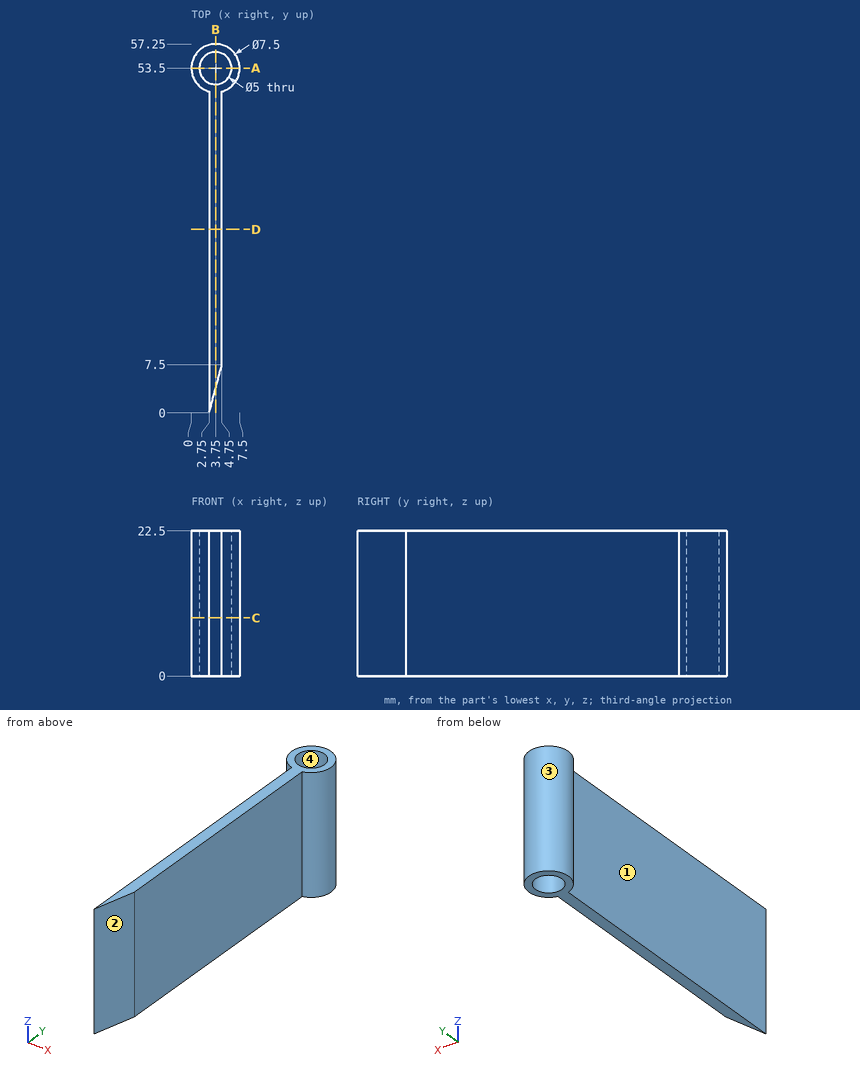
Print and shaded views of the part. All mm, measured from the part's lowest x, y and z. Round coordinates to 2 decimals unless told otherwise and drop trailing zeros. Write each loop counter-clockwise with the first axis right and the second up, starting at its lowest first coordinate (ties: lowest second). Pieces come first, ordered by that corner, then holes. Notation, with made-up numbers: (6.25, 67.25) - (40.25, 67.25) arc R23 ccw to (40.25, 98.25) - close; hole circle Ø5 at (0.5, 74.25). An arc over 180 degrees is marked (long way). Use CSV: the item, a comma, the result in double quotes. Start each with the question number.
Item 1: Two-plate mould, pull along Y, no slides. Class the marked faces 1, 2, 3 and 4: released by +Y, released by -Y, zero draft, split by the parting line, or undercut.
Item 2: Pin check, flat tips, straight feed: P1, Ø4, axis at y = 7, z = 18, coming from the +X side; P2, Ø1, axis at y = 29.5, z = 9.5, coming from the -X side; P3, Ø2, axis at y = 51.5, z = 3.5, coming from the -X side. Stop position of each tip, or through.
Item 3: Band-saw the part on D-D (y = 28.5). Write the cut outline in (x, z), and give its area (3 significant figures).
Item 4: Band-saw the part on C-C (z = 9). Write the cut outline in (x, y).
Item 5: Drill centre lines: L1, parallel to X at y = 48.5, z = 7; L2, parallel to Y at x = 2.5, z = 8; L3, parallel to Y at x = 5.75, z = 19.5. Where is each one in solid material? Low to high. Write a range as [from, to].
Item 6: Band-saw the part on B-B (x = 3.75). Write the cut outline in (y, z).
Item 7: Band-saw the part on A-A (y = 53.5). Write the cut outline in (x, z), and give its area (4 significant figures).
Checked values:
1,face 1,"zero draft"
1,face 2,"released by -Y"
1,face 3,"split by the parting line"
1,face 4,"undercut"
2,P1,"stops at x = 4.75"
2,P2,"stops at x = 2.75"
2,P3,"stops at x = 0.14"
3,outline,"(2.75, 0) - (4.75, 0) - (4.75, 22.5) - (2.75, 22.5) - close"
3,area,"45.0 mm²"
4,outline,"(2.75, 0) - (4.75, 7.5) - (4.75, 49.89) arc R3.75 ccw (long way) to (2.75, 49.89) - close; hole circle Ø5 at (3.75, 53.5)"
5,L1,"x = [2.75, 4.75]"
5,L2,"y = [49.96, 51.33], [55.67, 57.04]"
5,L3,"y = [50.33, 52], [55, 56.67]"
6,outline,"(3.75, 0) - (51, 0) - (51, 22.5) - (3.75, 22.5) - close; (56, 0) - (57.25, 0) - (57.25, 22.5) - (56, 22.5) - close"
7,outline,"(0, 0) - (1.25, 0) - (1.25, 22.5) - (0, 22.5) - close; (6.25, 0) - (7.5, 0) - (7.5, 22.5) - (6.25, 22.5) - close"
7,area,"56.25 mm²"
